For this review, take the finished solid that the model builds, in its own axes (mm). Face numbers are marked on the shaded views. A direction names the side the tool comes from. Round coordinates to 2 decimals unless told otherwise and drop trailing zeros.
1) Tool access review of the marked faces 1 and 2: name each direction out of +Z, -Z, +X, -X, +Y, -Y from which nothing blocks a thin tool from reaching the whole face with its end or side.
2) Wall thickness on L1, parallel to Y at x = 0, z = 1.4; L2, parallel to Z at x = 1, y = -1.5; L3, parallel to Z at x = -3.5, y = -0.5: over which ranges is each line inside the solid? List them lowest first.
3) Insertion check: pin 1 (2 mm diameter, centred on y = 2, z = 2, fed in from -X); pin 2 (3 mm diameter, centred on x = -2.5, z = 4, fed in from +Y); pin 3 (1.5 mm diameter, centred on x = -5, y = 3.5, fed in from -Z); pin 4 (4 mm diameter, centred on x = 1, y = -0.5, fed in from -Z). Each pin has a flat end and moves straight along its axis. Give the tip position at first contact, or say it passes through.
4) Mouldability with a two-part tool opening along X and no side actions: class the marked faces 3, 4, 5 and 6 as pulls with the +X half, pulls with the -X half, needs draft (parallel to the pull), parting line crosses it, or undercut.
```python
from build123d import *

# Parameters (mm, degrees)
F0_R     = 4
F1_DEPTH = 3
F2_R     = 6
F3_DEPTH = 8
F4_R     = 2.5
F5_DEPTH = 2
F6_R     = 1.99999
F7_R     = 2.5
F8_DEPTH = 2


# Not quite as in the source:
# - a fillet or chamfer is up to 0.001 mm smaller than in the source, because OpenCascade refuses the exact size


with BuildPart() as f1:
    # F0 (on Top) → F1 (new body)
    with BuildSketch(Plane.XY):
        Circle(F0_R)
    extrude(amount=F1_DEPTH)

    # F2 (on face) → F3 (join)
    with BuildSketch(Plane.XY.offset(3)):
        Circle(F2_R)
    extrude(amount=F3_DEPTH)

    # F4 (on face) → F5 (join)
    with BuildSketch(Plane.XY.offset(11)):
        Circle(F4_R)
    extrude(amount=F5_DEPTH)

    # F6 (radius 2 in the source; OpenCascade refuses exactly that, so slightly less here)
    f6_edges = [f1.edges().sort_by_distance(p)[0] for p in [
        (-6, 0, 11),
        (-6, 0, 3),
    ]]
    fillet(f6_edges, radius=F6_R)

    # F7 (on face) → F8 (cut)
    with BuildSketch(Plane(origin=(0, 0, 0), x_dir=(1, 0, 0), z_dir=(0, 0, -1))):
        Circle(F7_R)
    extrude(amount=-F8_DEPTH, mode=Mode.SUBTRACT)


solid = f1.part
```
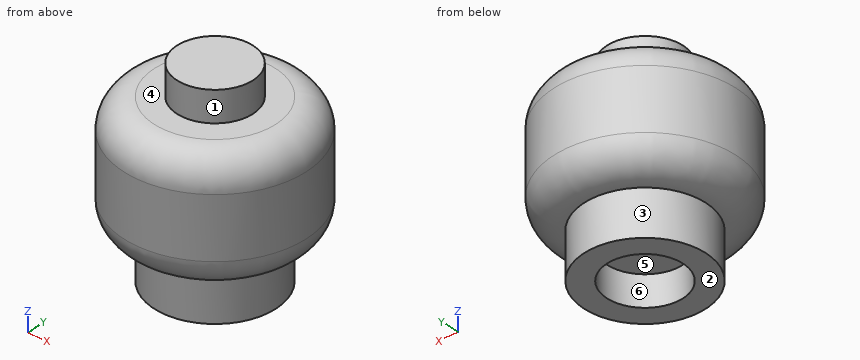
Response:
1. face 1: +Z
1. face 2: -Z, +X, -X, +Y, -Y
2. L1: y = -4 to -2.5, 2.5 to 4
2. L2: z = 2 to 13
2. L3: z = 0 to 11
3. pin 1: stops at x = -3.87
3. pin 2: stops at y = 5.86
3. pin 3: stops at z = 3.53
3. pin 4: stops at z = 0
4. face 3: parting line crosses it
4. face 4: needs draft
4. face 5: undercut
4. face 6: undercut
